Autodesk Inventor part; units mm, degrees
ref_plane "YZ Plane" through (0, 0, 0) normal (1, 0, 0) x (0, 1, 0)
ref_plane "XZ Plane" through (0, 0, 0) normal (0, 1, 0) x (-1, 0, 0)
ref_plane "XY Plane" through (0, 0, 0) normal (0, 0, 1) x (1, 0, 0)
ref_plane "Work Plane1" through (-0.0339, 0.0424, 0) normal (0, 0, 1) x (1, 0, 0)
sketch "Sketch1" plane through (-0.0339, 0.0424, 0) normal (0, 0, 1) x (1, 0, 0)
  circle A0 centre (-11, 0) radius 11
  circle A1 centre (-11, 0) radius 11.0762
  arc A2 (-22.1037, -29.7451) -> (-33.4506, 22.4506) centre (-11, 0) ccw
  line L0 (1.7, 12.7) -> (-23.7, 12.7)
  line L1 (-23.7, 12.7) -> (-23.7, -12.7)
  line L2 (-23.7, -12.7) -> (1.7, -12.7)
  line L3 (1.7, -12.7) -> (1.7, 12.7)
  line L4 (1.7, 12.7) -> (-23.7, -12.7) construction
  line L5 (-23.7, 12.7) -> (1.7, -12.7) construction
  circle A3 centre (8.05, 0) radius 2.1
  circle A4 centre (-11, 19.05) radius 2.1
  circle A5 centre (-30.05, 0) radius 2.1
  circle A6 centre (-11, -19.05) radius 2.1
  circle A7 centre (-11, 0) radius 14.2512
  circle A8 centre (-11, 0) radius 4.35
  line L6 (-33.4506, 22.4506) -> (-64.8815, -8.9803)
  arc A9 (-64.8815, -8.9803) -> (-63.7468, -14.1998) centre (-62.6365, -11.2253) ccw
  line L7 (-22.1037, -29.7451) -> (-63.7468, -14.1998)
  line L8 (-46.921, 8.9803) -> (-64.8815, -8.9803)
  point P0 (0.0339, -0.0424)
  point P1 (-23.7, 6.4658)
  point P2 (-17.4658, 12.7)
  point P3 (-17.4658, -12.7)
  point P4 (-23.7, -6.4658)
  point P5 (1.7, -6.4658)
  point P6 (-4.5342, -12.7)
  point P7 (-4.5342, 12.7)
  point P8 (1.7, 6.4658)
  point P9 (-42.4309, 4.4901)
  dimension "d0" = 0.0762
  dimension "d1" = 63.5
  dimension "d2" = 25.4
  dimension "d3" = 25.4
  dimension "d4" = 4.2
  dimension "d5" = 19.05
  dimension "d8" = 360
  dimension "d10" = 3.175
  dimension "d15" = 8.7
  dimension "d23" = 6.35
extrude "Extrusion1" add sketch "Sketch1" along normal blind 16.505 contours A7 L3 L2 L1 L0 | L0 A7 | A7 L3 | L1 A7 | A7 L2
extrude "Extrusion2" add sketch "Sketch1" along normal blind 9.525 contours L7 A9 L6 A2 | L3 A7 L0 | A7 L3 L2 L1 L0 | L0 A7 | A7 L3 | A7 L1 L0 | L3 L2 A7 | L1 A7 | A7 L2 | A7 L2 L1
extrude "Extrusion3" add sketch "Sketch1" along normal blind 2.505 contours A0 | A1
extrude "Extrusion4" add sketch "Sketch1" along normal blind 13.97 contours L3 A7 L0 | A7 L1 L0 | L3 L2 A7 | A7 L2 L1
chamfer "Chamfer1" distance 0.635 angle 45 14 edges at (-22.1101, 0.0424, 16.505) (5.9161, 0.0424, 9.525) (-13.1339, 19.0924, 9.525) (-13.1339, -19.0076, 9.525) (-32.1839, 0.0424, 9.525) (1.6661, 9.6253, 13.97) (-1.451, 12.7424, 13.97) (-20.6168, 12.7424, 13.97) (-23.7339, 9.6253, 13.97) (1.6661, -9.5405, 13.97) (-1.451, -12.6576, 13.97) (-23.7339, -9.5405, 13.97) (-20.6168, -12.6576, 13.97) (-25.2851, 0.0424, 16.505)
properties part number "WeightBearingMount"
Geometry: final body of the model. Coordinates: model frame, mm. A direction names the side the tool comes from. Coordinates: 2 decimals unless noted, no trailing zeros. Order: outer loops, then holes, each group sorted by start corner. A loop starts at its lowest first (then second) coordinate and runs counter-clockwise, first axis right, second up. Notation, with made-up numbers: M 58.25,75 L 85.25,75 A34 cw 85.25,114 Z; hole C -25.5,11 d2. An arc over 180 degrees is marked long. Answer in a Markdown table with one row per item. Add a question column.
Q1. Section query A-A on z = 6.5. Return the cut outline in (x, y).
Q2. Contact query for flat-ended pins moving along their axis: P1, Ø6.5, axis at x = -14.5, y = -0.5, coming from the +Z side (3 decimals); P2, Ø1.1, axis at y = -9.5, z = 12, coming from the -X side; P3, Ø3.5, axis at x = -11.03, y = -19.01, coming from the -Z side; P4, Ø8, axis at x = -31, z = 11, coming from the -Y side. Output: stop coordinate, or through.
Q3. Reachability of faces 1 (the cylindrical face through (-13.435, 10.855, 9.094)), 2 (the flat face through (-1, -12.658, 11)), 3 (the flat face through (-23.734, 10, 11)), 4 (the flat face through (0, 11, 13.97)) from +Z, -Z, +X, -X, +Y, -Y: full face, straight path, thin tool, end or side. Return the list, or none.
Q4. Section query C-C on x = -36. Return the cut outline in (y, z) (1 decimal), and give its area (3 significant figures).
Q5. Section query D-D on y = -23. Return the cut outline in (x, z) (3 decimals), and give its area (3 significant figures).
Q6. Line query: L1, parallel to Y at x = -9.5, z = 4; L2, parallel to Z at x = -26, y = 6.5 (3 decimals); L3, parallel to Y at x = -8, z = 13. Output: solid intervals per line, ascending.
Q7. Section query B-B on z = 12.25. Return the cut outline in (x, y), and give its area (3 significant figures).
Completed:
| question | item | result |
|---|---|---|
| 1 | outline | M -64.92,-8.94 A3.17 ccw -63.78,-14.16 L -22.14,-29.7 A31.75 ccw long -33.48,22.49 Z; hole C -30.08,0.04 d4.2; hole C -11.03,0.04 d22.15; hole C -11.03,-19.01 d4.2; hole C -11.03,19.09 d4.2; hole C 8.02,0.04 d4.2 |
| 2 | P1 | stops at z = 2.505 |
| 2 | P2 | stops at x = -23.73 |
| 2 | P3 | passes through |
| 2 | P4 | stops at y = -27.78 |
| 3 | face 1 | +Z |
| 3 | face 2 | +Z, +X, -Y |
| 3 | face 3 | +Z, -X, +Y |
| 3 | face 4 | +Z, +X, +Y |
| 4 | outline | M -24.5,0 L 20,0 L 20,9.5 L -24.5,9.5 Z |
| 4 | area | 424 mm2 |
| 5 | outline | M -40.093,0 L 10.809,0 L 10.809,9.525 L -40.093,9.525 Z |
| 5 | area | 485 mm2 |
| 6 | L1 | y = -31.67 to -20.44, -17.57 to -10.93, 11.01 to 17.66, 20.53 to 31.76 |
| 6 | L2 | z = 0 to 9.525 |
| 6 | L3 | y = -13.88 to -10.61, 10.69 to 13.97 |
| 7 | outline | M -23.73,-12.66 L -17.5,-12.66 A14.25 ccw -4.57,-12.66 L 1.67,-12.66 L 1.67,-6.42 A14.25 ccw 1.67,6.51 L 1.67,12.74 L -4.57,12.74 A14.25 ccw -17.5,12.74 L -23.73,12.74 L -23.73,6.51 A14.25 ccw -23.73,-6.42 Z; hole C -11.03,0.04 d22.15 |
| 7 | area | 314 mm2 |
